from build123d import *

# Parameters (mm, degrees)
F0_W      = 30
F0_H      = 30
F2_W      = 35
F2_H      = 35
F4_R      = 16.5
F5_R      = 14
F7_R      = 1.25
F8_DEPTH  = 2
F9_R      = 1.5
F10_DEPTH = 5


with BuildPart() as f3:
    # F0 (on Top) → F3 section 0
    with BuildSketch(Plane.XY):
        with Locations((15, -15)):
            Rectangle(F0_W, F0_H)
    # F2 (on offset) → F3 section 1
    with BuildSketch(Plane.XY.offset(5)):
        with Locations((15, -15)):
            Rectangle(F2_W, F2_H)
    loft()

    # F4 (on face) → F6 section 0
    with BuildSketch(Plane.XY.offset(5)):
        with Locations((15, -15)):
            Circle(F4_R)
    # F5 (on face) → F6 section 1
    with BuildSketch(Plane(origin=(0, 0, 0), x_dir=(1, 0, 0), z_dir=(0, 0, -1))):
        with Locations((15, 15)):
            Circle(F5_R)
    loft(mode=Mode.SUBTRACT)

    # F7 (on face) → F8 (join)
    with BuildSketch(Plane.XY.offset(5)):
        with Locations((0.5, -0.5)):
            Circle(F7_R)
        with Locations((29.5, -0.5)):
            Circle(F7_R)
        with Locations((29.5, -29.5)):
            Circle(F7_R)
        with Locations((0.5, -29.5)):
            Circle(F7_R)
    extrude(amount=F8_DEPTH)

    # F9 (on face) → F10 (cut)
    with BuildSketch(Plane.XY):
        with Locations((27, -27)):
            Circle(F9_R)
        with Locations((3, -27)):
            Circle(F9_R)
        with Locations((3, -3)):
            Circle(F9_R)
        with Locations((27, -3)):
            Circle(F9_R)
    extrude(amount=F10_DEPTH, mode=Mode.SUBTRACT)


solid = f3.part
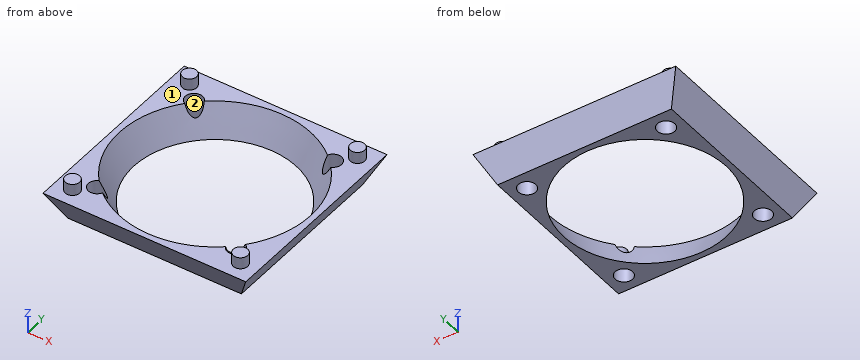
Here's how the part is built. I have some questions about the finished solid (model axes, mm). Face numbers are marked on the shaded views. A direction names the side the tool comes from. Round coordinates to 2 decimals unless told otherwise and drop trailing zeros. Write each question's results on one line, items separated by ' | '.
(1) If I drill on L1, parallel to Y at x = 3, z = 1.75 (3 decimals); L2, parallel to Y at x = 27, z = 2.25 (3 decimals); L3, parallel to X at y = -3, z = 3, over which ranges is the centre line in solid material (lowest first)?
Worked answers:
L1: -30.875 to -28.5, -25.5 to -23.79, -6.21 to -4.5, -1.5 to 0.875 | L2: -31.125 to -28.5, -25.5 to -24.207, -5.793 to -4.5, -1.5 to 1.125 | L3: -1.5 to 1.5, 4.5 to 5.19, 24.81 to 25.5, 28.5 to 31.5
(2) For P1, Ø8, axis at x = 26, y = -14, coming from the +Z side; P2, Ø17.5, axis at x = 23, y = -13.5, coming from the +Z side; P3, Ø4, axis at y = -9, z = 1.5, coming from the +X side; P4, Ø2.5, axis at x = 27, y = -27, coming from the -Z side, each with a flat end and sliding along its axis, tell me the tip position at first contact or that it passes through.
Worked answers:
P1: z = 2.09 | P2: z = 5 | P3: x = 31.75 | P4: through
(3) For the marked faces 1 and 2, which set-ups out of +Z, -Z, +X, -X, +Y, -Y let a thin tool reach every point of the face, with its end or its side?
Worked answers:
face 1: +Z | face 2: +Z, -Z
(4) If we section it at A-A, the plane z = 1.25: Give the number of separate pieces and of enclosed holes in the cut face, then the cut area to 3 significant figures.
Worked answers:
separate pieces: 1 | enclosed holes: 5 | area: 276 mm2
